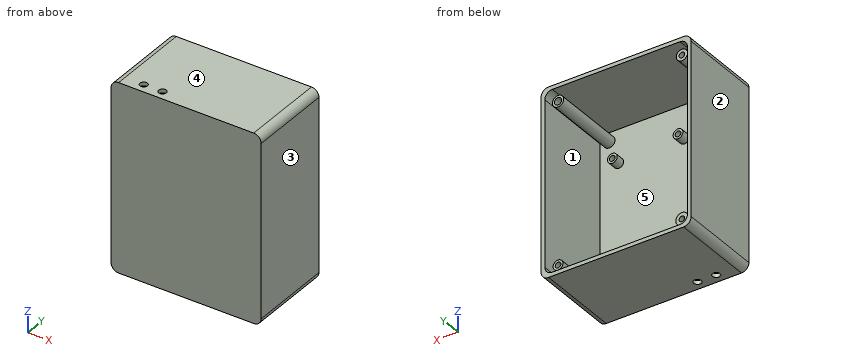
```python
from build123d import *

# Parameters (mm, degrees)
SKETCH1_W            = 80
SKETCH1_H            = 100
BOSS_EXTRUDE1_DEPTH  = 45
SHELL1_T             = -2
FILLET1_R            = 4
FILLET2_R            = 4
FILLET4_R            = 4
FILLET5_R            = 4
FILLET6_R            = 4
FILLET7_R            = 4
FILLET12_R           = 4
FILLET13_R           = 4
SKETCH33_R           = 2.6
BOSS_EXTRUDE9_DEPTH  = 5
SKETCH37_R           = 2.624374832
SKETCH37_R_2         = 3
SKETCH37_R_3         = 3.264262679
BOSS_EXTRUDE10_DEPTH = 40
SKETCH38_R           = 1.5
SKETCH38_R_2         = 1.938271083
CUT_EXTRUDE3_DEPTH   = 40
SKETCH39_R           = 1.5
CUT_EXTRUDE4_DEPTH   = 5
SKETCH40_R           = 2
CUT_EXTRUDE5_DEPTH   = 10
CUT_EXTRUDE6_START   = -10
SKETCH41_R           = 2
CUT_EXTRUDE6_DEPTH   = 10


with BuildPart() as part:
    # Sketch1 → Boss-Extrude1 (new body)
    with BuildSketch(Plane(origin=(0, 0, 0), x_dir=(1, 0, 0), z_dir=(0, 1, 0))):
        Rectangle(SKETCH1_W, SKETCH1_H)
    extrude(amount=BOSS_EXTRUDE1_DEPTH)

    # Shell1
    shell1_openings = [part.faces().sort_by_distance(p)[0] for p in [
        (0, 45, 0),
    ]]
    offset(amount=SHELL1_T, openings=shell1_openings, kind=Kind.INTERSECTION)

    # Fillet1
    fillet1_edges = [part.edges().sort_by_distance(p)[0] for p in [
        (-40, 22.5, 50),
    ]]
    fillet(fillet1_edges, radius=FILLET1_R)

    # Fillet2
    fillet2_edges = [part.edges().sort_by_distance(p)[0] for p in [
        (-38, 23.5, 48),
    ]]
    fillet(fillet2_edges, radius=FILLET2_R)

    # Fillet4
    fillet4_edges = [part.edges().sort_by_distance(p)[0] for p in [
        (-38, 23.5, -48),
    ]]
    fillet(fillet4_edges, radius=FILLET4_R)

    # Fillet5
    fillet5_edges = [part.edges().sort_by_distance(p)[0] for p in [
        (-40, 22.5, -50),
    ]]
    fillet(fillet5_edges, radius=FILLET5_R)

    # Fillet6
    fillet6_edges = [part.edges().sort_by_distance(p)[0] for p in [
        (38, 23.5, 48),
    ]]
    fillet(fillet6_edges, radius=FILLET6_R)

    # Fillet7
    fillet7_edges = [part.edges().sort_by_distance(p)[0] for p in [
        (40, 22.5, 50),
    ]]
    fillet(fillet7_edges, radius=FILLET7_R)

    # Fillet12
    fillet12_edges = [part.edges().sort_by_distance(p)[0] for p in [
        (40, 22.5, -50),
    ]]
    fillet(fillet12_edges, radius=FILLET12_R)

    # Fillet13
    fillet13_edges = [part.edges().sort_by_distance(p)[0] for p in [
        (38, 23.5, -48),
    ]]
    fillet(fillet13_edges, radius=FILLET13_R)

    # Sketch33 → Boss-Extrude9 (add)
    with BuildSketch(Plane(origin=(0, 2, 0), x_dir=(1, 0, 0), z_dir=(0, 1, 0))):
        with Locations(Location((28, 30, 0), (0, 0, 270))):
            Circle(SKETCH33_R)
        with Locations(Location((28, -30, 0), (0, 0, 270))):
            Circle(SKETCH33_R)
        with Locations(Location((-7, 30, 0), (0, 0, 270))):
            Circle(SKETCH33_R)
        with Locations(Location((-7, -30, 0), (0, 0, 270))):
            Circle(SKETCH33_R)
    extrude(amount=BOSS_EXTRUDE9_DEPTH)

    # Sketch37 → Boss-Extrude10 (add)
    with BuildSketch(Plane(origin=(0, 2, 0), x_dir=(1, 0, 0), z_dir=(0, 1, 0))):
        with Locations(Location((33, 43, 0), (0, 0, 270))):
            Circle(SKETCH37_R)
        with Locations(Location((33, -43, 0), (0, 0, 270))):
            Circle(SKETCH37_R_2)
        with Locations(Location((-33, 43, 0), (0, 0, 270))):
            Circle(SKETCH37_R_3)
        with Locations(Location((-33, -43, 0), (0, 0, 270))):
            Circle(SKETCH37_R_2)
    extrude(amount=BOSS_EXTRUDE10_DEPTH)

    # Sketch38 → Cut-Extrude3 (cut)
    with BuildSketch(Plane(origin=(0, 42, 0), x_dir=(1, 0, 0), z_dir=(0, 1, 0))):
        with Locations(Location((33, 43, 0), (0, 0, 270))):
            Circle(SKETCH38_R)
        with Locations(Location((33, -43, 0), (0, 0, 270))):
            Circle(SKETCH38_R_2)
        with Locations(Location((-33, 43, 0), (0, 0, 270))):
            Circle(SKETCH38_R)
        with Locations(Location((-33, -43, 0), (0, 0, 270))):
            Circle(SKETCH38_R)
    extrude(amount=-CUT_EXTRUDE3_DEPTH, mode=Mode.SUBTRACT)

    # Sketch39 → Cut-Extrude4 (cut)
    with BuildSketch(Plane(origin=(0, 7, 0), x_dir=(1, 0, 0), z_dir=(0, 1, 0))):
        with Locations(Location((28, 30, 0), (0, 0, 270))):
            Circle(SKETCH39_R)
        with Locations(Location((28, -30, 0), (0, 0, 270))):
            Circle(SKETCH39_R)
        with Locations(Location((-7, 30, 0), (0, 0, 270))):
            Circle(SKETCH39_R)
        with Locations(Location((-7, -30, 0), (0, 0, 270))):
            Circle(SKETCH39_R)
    extrude(amount=-CUT_EXTRUDE4_DEPTH, mode=Mode.SUBTRACT)

    # Sketch40 → Cut-Extrude5 (cut)
    with BuildSketch(Plane.XY.offset(50)):
        with Locations((-26, 5)):
            Circle(SKETCH40_R)
        with Locations((-16, 5)):
            Circle(SKETCH40_R)
    extrude(amount=-CUT_EXTRUDE5_DEPTH, mode=Mode.SUBTRACT)

    # Sketch41 → Cut-Extrude6 (cut)
    with BuildSketch(Plane(origin=(0, 0, -50), x_dir=(-1, 0, 0), z_dir=(0, 0, -1)).offset(CUT_EXTRUDE6_START)):
        with Locations(Location((26, 5, 0), (0, 0, 180))):
            Circle(SKETCH41_R)
        with Locations(Location((16, 5, 0), (0, 0, 180))):
            Circle(SKETCH41_R)
    extrude(amount=CUT_EXTRUDE6_DEPTH, mode=Mode.SUBTRACT)


solid = part.part
```
Part model, mm, in its own coordinate system. Face numbers are marked on the shaded views. A direction names the side the tool comes from. Coordinates: 2 decimals unless noted, no trailing zeros. Write each loop counter-clockwise with the first axis right and the second up, starting at its lowest first coordinate (ties: lowest second). Pieces come first, ordered by that corner, then holes.
Item 1: Which spindle directions (+Z, -Z, +X, -X, +Y, -Y) get a long thin tool onto all of the face, cutting with end or side? Do the marked faces 1 and 2. Say none if no direction does.
Item 2: Slice it at C-C (z = 30). Write the cut outline in (x, y).
Item 3: Probe line 1 (X direction, y = 4.5, z = -30); line 2 (X direction, y = 40, z = -34); line 3 (Z direction, x = -8, y = 15). List the from-to ranges inside material, lowest first.
Item 4: Mould opens along X. For the marked faces 3, 4 and 5 say: released by +X, released by -X, zero draft, split by the parting line, or undercut.
Item 5: Slice it at B-B (x = -7). Write the cut outline in (y, z), and give its area (3 significant figures).
Item 6: Slice it at A-A (y = 20.5). Count the separate pieces of the cut face and the enclosed holes in it, and give its area (3 significant figures).
Item 7: Pin check, flat tips, straight feed: pin 1 (5 mm diameter, centred on x = -33, z = -43, fed in from +Y); pin 2 (2.5 mm diameter, centred on x = -7.5, z = -30.5, fed in from +Y). Stop position of each tip, or through.
Results found:
1. face 1: +Y
1. face 2: +Z, -Z, -X, +Y, -Y
2. outline: (-40, 0) - (40, 0) - (40, 45) - (38, 45) - (38, 2) - (30.6, 2) - (30.6, 7) - (29.5, 7) - (29.5, 2) - (26.5, 2) - (26.5, 7) - (25.4, 7) - (25.4, 2) - (-4.4, 2) - (-4.4, 7) - (-5.5, 7) - (-5.5, 2) - (-8.5, 2) - (-8.5, 7) - (-9.6, 7) - (-9.6, 2) - (-38, 2) - (-38, 45) - (-40, 45) - close
3. line 1: x = -40 to -38, -9.6 to -8.5, -5.5 to -4.4, 25.4 to 26.5, 29.5 to 30.6, 38 to 40
3. line 2: x = -40 to -38, 38 to 40
3. line 3: z = -50 to -48, 48 to 50
4. face 3: released by +X
4. face 4: zero draft
4. face 5: undercut
5. outline: (0, -50) - (45, -50) - (45, -48) - (2, -48) - (2, -32.6) - (7, -32.6) - (7, -31.5) - (2, -31.5) - (2, -28.5) - (7, -28.5) - (7, -27.4) - (2, -27.4) - (2, 27.4) - (7, 27.4) - (7, 28.5) - (2, 28.5) - (2, 31.5) - (7, 31.5) - (7, 32.6) - (2, 32.6) - (2, 48) - (45, 48) - (45, 50) - (0, 50) - close
5. area: 394 mm2
6. separate pieces: 5
6. enclosed holes: 5
6. area: 783 mm2
7. pin 1: stops at y = 42
7. pin 2: stops at y = 7
